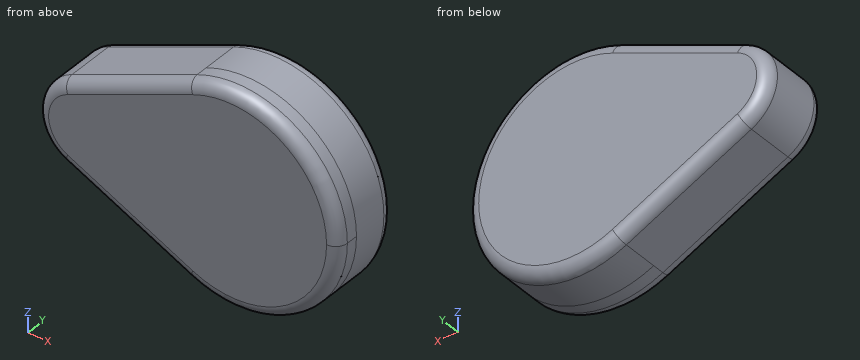
```python
from build123d import *

# Parameters (mm, degrees)
F1_DEPTH = 25.4
F2_R     = 57.300749
F3_DEPTH = 25.4
F4_DEPTH = 50.8
F5_R     = 12.7
F6_R     = 12.7


with BuildPart() as f1:
    # F0 (on Front) → F1 (new body)
    with BuildSketch(Plane.XZ):
        with BuildLine():
            ThreePointArc((-84.642182, -43.85329), (-38.706084, -40.44707), (-16.666076, 0))
            ThreePointArc((-16.666076, 0), (-38.706084, 40.44707), (-84.642182, 43.85329))
            ThreePointArc((-84.642182, 43.85329), (-112.933167, 0), (-84.642182, -43.85329))
        make_face()
        with BuildLine():
            ThreePointArc((51.31003, -105.3684), (1.802586, -62.696194), (-16.666076, 0))
            ThreePointArc((-16.666076, 0), (-38.706084, -40.44707), (-84.642182, -43.85329))
            Line((-84.642182, -43.85329), (51.31003, -105.3684))
        make_face()
        with BuildLine():
            ThreePointArc((-84.642182, 43.85329), (-38.706084, 40.44707), (-16.666076, 0))
            ThreePointArc((-16.666076, 0), (1.802586, 62.696194), (51.31003, 105.3684))
            Line((51.31003, 105.3684), (-84.642182, 43.85329))
        make_face()
        with BuildLine():
            ThreePointArc((51.31003, 105.3684), (1.802586, 62.696194), (-16.666076, 0))
            ThreePointArc((-16.666076, 0), (1.802586, -62.696194), (51.31003, -105.3684))
            ThreePointArc((51.31003, -105.3684), (161.682894, -97.184114), (214.639476, 0))
            ThreePointArc((214.639476, 0), (161.682894, 97.184114), (51.31003, 105.3684))
        make_face()
    extrude(amount=F1_DEPTH)

    # F2 (on Front) → F3 (cut)
    with BuildSketch(Plane.XZ):
        with Locations((105.685264, 0)):
            Circle(F2_R)
    extrude(amount=-F3_DEPTH, mode=Mode.SUBTRACT)

    # F1_face (on face) → F4 (join)
    with BuildSketch(Plane(origin=(66.909918, 0, 0), x_dir=(1, 0, 0), z_dir=(0, 1, 0))):
        with BuildLine():
            ThreePointArc((-151.5521, 43.85329), (-179.843085, 0), (-151.5521, -43.85329))
            Line((-151.5521, -43.85329), (-15.599888, -105.3684))
            ThreePointArc((-15.599888, -105.3684), (147.729558, 0), (-15.599888, 105.3684))
            Line((-15.599888, 105.3684), (-151.5521, 43.85329))
        make_face()
    extrude(amount=F4_DEPTH)

    # F5
    f5_edges = [f1.edges().sort_by_distance(p)[0] for p in [
        (-16.666076, 50.8, 74.610845),
    ]]
    fillet(f5_edges, radius=F5_R)

    # F6
    f6_edges = [f1.edges().sort_by_distance(p)[0] for p in [
        (-16.666076, -25.4, 74.610845),
    ]]
    fillet(f6_edges, radius=F6_R)


solid = f1.part
```
Work out the finished part from the listing and answer in its coordinate system (mm). Give positions to 0.01 mm unless a question says otherwise; leave off trailing zeros. Loops run counter-clockwise (first coordinate to the right, second up) from the corner with the lowest first, then second, coordinate; pieces in that order, holes last. Notation, with made-up numbers: (-3, 67.5) -> (14, 67.5) arc R19 ccw to (14, 76.5) -> close; hole circle Ø9 at (12.25, -13.75). An arc over 180 degrees is marked (long way). Put each result on its own line as item: value. Start each with the question number.
Item 1: The part is cut by section A-A (y = -20). Give the vertices of the cut face in (x, z), then the cut area to 3 significant figures.
Item 2: Each of these flat-tipped pins is pushed along its axis until it touches: P1, Ø3, axis at x = 47, y = -12, coming from the -Z side; P2, Ø5, axis at y = 43, z = -68.5, coming from the +X side; P3, Ø1.5, axis at x = -10.5, z = -67.5, coming from the -Y side. Where does it stop, or does it pass through?
Item 3: Find the intervals of material crossed by L1, parallel to X at y = 40.5, z = -29; L2, parallel to X at y = 46, z = 97; L3, parallel to Z at x = 125, y = 15.5, in increasing order. Write a range as [from, to].
Answers below:
1. outline: (-83.69, -41.75) -> (52.26, -103.27) arc R113.35 ccw to (212.33, 0) arc R113.35 ccw to (52.26, 103.27) -> (-83.69, 41.75) arc R45.83 ccw to start
1. area: 51,800 mm2
2. P1: z = -104.1
2. P2: x = 193.07
2. P3: y = -25.06
3. L1: [-102.93, 210.71]
3. L2: [39.5, 156.75]
3. L3: [-112.69, 112.69]
